from build123d import *

# Parameters (mm, degrees)
F0_W     = 43.688
F0_H     = 43.688
F0_R     = 9.652
F1_DEPTH = 43.688
F2_R     = 9.652
F3_DEPTH = 43.689
F4_R     = 9.652
F5_DEPTH = 43.689


with BuildPart() as f1:
    # F0 (on Front) → F1 (new body)
    with BuildSketch(Plane.XZ):
        with Locations((-21.844, 21.844)):
            Rectangle(F0_W, F0_H)
        with Locations((-21.844, 21.844)):
            Circle(F0_R, mode=Mode.SUBTRACT)
    extrude(amount=F1_DEPTH)

    # F2 (on face) → F3 (cut, through all)
    with BuildSketch(Plane(origin=(0, 0, 0), x_dir=(1, 0, 0), z_dir=(0, 0, -1))):
        with Locations((-21.844, 21.844)):
            Circle(F2_R)
    extrude(amount=-F3_DEPTH, mode=Mode.SUBTRACT)

    # F4 (on Right) → F5 (cut, through all)
    with BuildSketch(Plane.YZ):
        with Locations((-21.844, 21.844)):
            Circle(F4_R)
    extrude(amount=-F5_DEPTH, mode=Mode.SUBTRACT)


solid = f1.part
Model file for the job. Use its own axes, mm. Round coordinates to 2 decimals unless told otherwise and drop trailing zeros. Order: outer loops, then holes, each group sorted by start corner. A loop starts at its lowest first (then second) coordinate and runs counter-clockwise, first axis right, second up.
(1) Pin check, flat tip, straight feed: pin 1 (11.5 mm diameter, centred on y = -21.844, z = 21.844, fed in from +X). Stop position of the tip, or through.
(2) Band-saw the part on B-B (x = -16.5). List the corners of the cut face in (y, z).
(3) Band-saw the part on D-D (y = -10.5). List the corners of the cut face in (x, z), then the cut area to 3 significant figures.
(4) Band-saw the part on A-A (y = -20). List the corners of the cut face in (x, z).
(5) Drill centre lines: line 1 (Y direction, x = -8, z = 30); line 2 (Z direction, x = -15, y = -41); line 3 (Y direction, x = -7.5, z = 25.5). Where is each one in solid material? Low to high.
(6) Pull direction X, two halves, no side cores. Call faces 1 (the face through (0, -12, 22)), 2 (the face through (-23.936, -12.422, 7.404)), 3 (the face through (-32, -22, 0)): released by +X, released by -X, zero draft, split by the parting line, or undercut.
(7) Band-saw the part on C-C (z = 11.5). List the corners of the cut face in (x, y), then the cut area to 3 significant figures.
Verdict:
1. pin 1: passes through
2. outline: (-43.69, 0) - (-29.88, 0) - (-29.88, 13.81) - (-43.69, 13.81) - close; (-43.69, 29.88) - (-29.88, 29.88) - (-29.88, 43.69) - (-43.69, 43.69) - close; (-13.81, 0) - (0, 0) - (0, 13.81) - (-13.81, 13.81) - close; (-13.81, 29.88) - (0, 29.88) - (0, 43.69) - (-13.81, 43.69) - close
3. outline: (-43.69, 0) - (0, 0) - (0, 43.69) - (-43.69, 43.69) - close; hole circle Ø19.3 at (-21.84, 21.84)
3. area: 1,620 mm2
4. outline: (-43.69, 0) - (-31.32, 0) - (-31.32, 12.37) - (-43.69, 12.37) - close; (-43.69, 31.32) - (-31.32, 31.32) - (-31.32, 43.69) - (-43.69, 43.69) - close; (-12.37, 0) - (0, 0) - (0, 12.37) - (-12.37, 12.37) - close; (-12.37, 31.32) - (0, 31.32) - (0, 43.69) - (-12.37, 43.69) - close
5. line 1: y = -43.69 to -27.01, -16.68 to 0
5. line 2: z = 0 to 15.04, 28.65 to 43.69
5. line 3: y = -43.69 to -30.78, -12.91 to 0
6. face 1: released by +X
6. face 2: undercut
6. face 3: zero draft
7. outline: (-43.69, -43.69) - (0, -43.69) - (0, 0) - (-43.69, 0) - close; hole circle Ø19.3 at (-21.84, -21.84)
7. area: 1,620 mm2
